Could you check a few things on this model? Use its own coordinates, in mm. A direction names the side the tool comes from. Coordinates: 2 decimals unless noted, no trailing zeros. Loops run counter-clockwise (first coordinate to the right, second up) from the corner with the lowest first, then second, coordinate; pieces in that order, holes last.
1) Imagine slicing it at A-A on x = 0. Please give me the cut outline in (y, z).
2) Will these pins go through, and if not, where does the flat tip stop? P1, Ø3, axis at x = -8, z = 3.5, coming from the -Y side; P2, Ø0.5, axis at y = 0.5, z = 2, coming from the -X side; P3, Ø1.9, axis at x = -11.5, z = 1.5, coming from the -Y side.
3) If I drill on line 1 along Y through (x, z) = (-10.5, 3.1); line 2 along Y through (x, z) = (0, 1.7); line 3 along Z through (x, y) = (16, -1), over which ranges is the centre line in solid material (lowest first)?
4) Imagine slicing it at B-B on x = -10.5. Please give me the cut outline in (y, z), plus the area to 3 significant figures.
5) Thinking about a two-plate mould opening in X: for faces 6 (the face through (8, -3, 5)), 7 (the face through (-9, 1, 2)), 8 (the face through (5.58, 0.1, 2.46)), which applies, released by +X, released by -X, zero draft, split by the parting line, or undercut?
6) For faces 1 (the face through (-7, 0, 2)), 2 (the face through (4.883, -1.928, 3.732)), 3 (the face through (-4.19, 3.16, 3.73)), 4 (the face through (7.98, -0.36, 2.46)), 5 (the face through (3.44, -4.82, 2.46)), which set-ups out of +Z, -Z, +X, -X, +Y, -Y let a thin tool reach every point of the face, with its end or its side?
```python
from build123d import *

# Parameters (mm, degrees)
SKETCH1_R               = 1.5
BOSS_EXTRUDE1_DEPTH     = 5
BOSS_EXTRUDE1_2_DEPTH   = 5
SKETCH1_3_R             = 5.25
BOSS_EXTRUDE2_DEPTH     = 2.5
CUT_EXTRUDE4_DEPTH      = 34.791042337
CUT_EXTRUDE4_DEPTH_BACK = 34.791042337
SKETCH1_5_R             = 3.25
CUT_EXTRUDE1_DEPTH      = 34.791042337
CUT_EXTRUDE2_DEPTH      = 34.791042337
LPATTERN1_COUNT         = 28
LPATTERN1_PITCH         = 0.5
CUT_EXTRUDE3_DEPTH      = 34.791042337
CIRPATTERN1_COUNT       = 8
CIRPATTERN1_ANGLE       = 42


with BuildPart() as part:
    # Sketch1 → Boss-Extrude1 (new body)
    with BuildSketch(Plane.XY):
        with BuildLine():
            Line((-1.559459186, 5.819980914), (-9.630372069, 7.89024295))
            ThreePointArc((-9.630372069, 7.89024295), (-13.619847961, 6.086363356), (-12.727105745, 1.8))
            Line((-12.727105745, 1.8), (-9, 1.8))
            Line((-9, 1.8), (-9, 0))
            Line((-9, 0), (-5.25, 0))
            ThreePointArc((-5.25, 0), (-4.165105037, 3.195997502), (-1.358799987, 5.071110588))
            Line((-1.358799987, 5.071110588), (-1.559459186, 5.819980914))
        make_face()
        with Locations((-10.5, 4.5)):
            Circle(SKETCH1_R, mode=Mode.SUBTRACT)
    extrude(amount=BOSS_EXTRUDE1_DEPTH)



with BuildPart() as body_2:
    # Sketch1 → Boss-Extrude1 2 (new body)
    with BuildSketch(Plane.XY):
        with BuildLine():
            Line((5.983025461, -0.728942102), (5.162088265, 0.956736509))
            ThreePointArc((5.162088265, 0.956736509), (4.867715236, -1.966684615), (3.048690517, -4.274106471))
            Line((3.048690517, -4.274106471), (3.844408913, -5.389662519))
            Line((3.844408913, -5.389662519), (13.676957988, -3.567307264))
            Line((13.676957988, -3.567307264), (32.08570782, 4.250488438))
            Line((32.08570782, 4.250488438), (32.44741195, 6.013772341))
            Line((32.44741195, 6.013772341), (18.681843244, 3.462474984))
            ThreePointArc((18.681843244, 3.462474984), (14.653100202, 0.834635979), (9.916045092, 0))
            Line((9.916045092, 0), (5.983025461, -0.728942102))
        make_face()
    extrude(amount=BOSS_EXTRUDE1_2_DEPTH)


with BuildPart() as part_1:
    add(part.part)

    add(body_2.part)  # Boss-Extrude2 merges body 2
    # Sketch1<3> → Boss-Extrude2 (add)
    with BuildSketch(Plane.XY):
        Circle(SKETCH1_3_R)
    extrude(amount=BOSS_EXTRUDE2_DEPTH)

    # Sketch1<5> → Cut-Extrude4 (cut, two sides: drawn at the far end of the back side and taken through both)
    with BuildSketch(Plane.XY.offset(-CUT_EXTRUDE4_DEPTH_BACK)):
        Circle(SKETCH1_5_R)
    extrude(amount=CUT_EXTRUDE4_DEPTH + CUT_EXTRUDE4_DEPTH_BACK, mode=Mode.SUBTRACT)

    # Sketch2 → Cut-Extrude1 (cut, through all)
    with BuildSketch(Plane(origin=(0, 0, 0), x_dir=(0.9832549075639557, 0.18223552549214142, 0), z_dir=(-0.18223552549214142, 0.9832549075639557, 0))):
        Polygon((13, 0), (33, -1.875), (33, 0), align=None)
        Polygon((33, -3.125), (33, -5), (13, -5), align=None)
    extrude(amount=-CUT_EXTRUDE1_DEPTH, mode=Mode.SUBTRACT)

    # Sketch3 → Cut-Extrude2 (cut, symmetric)
    with BuildSketch(Plane.XY):
        Polygon((31.759133514, 5.886207473), (32.03228257, 5.784278119), (32.250760968, 5.977325236), align=None)
    cut_extrude2 = extrude(amount=CUT_EXTRUDE2_DEPTH, both=True, mode=Mode.SUBTRACT)

    # LPattern1: Cut-Extrude2 ×28
    with Locations(*[Vector(-0.983254907563956, -0.1822355254921403, 0) * (i * LPATTERN1_PITCH) for i in range(1, LPATTERN1_COUNT)]):
        add(cut_extrude2, mode=Mode.SUBTRACT)

    # Sketch4 → Cut-Extrude3 (cut, through all)
    with BuildSketch(Plane.XY):
        Polygon((9.916045092, 0), (11.165663009, 0.030904073), (10.553215679, -0.48439513), align=None)
    cut_extrude3 = extrude(amount=CUT_EXTRUDE3_DEPTH, mode=Mode.SUBTRACT)

    # CirPattern1: Cut-Extrude3 ×8 about axis
    cirpattern1_axis = Axis((10.244577616, 11.995501923, 0), (0, 0, 1))
    for i in range(1, CIRPATTERN1_COUNT):
        add(cut_extrude3.rotate(cirpattern1_axis, i * CIRPATTERN1_ANGLE / (CIRPATTERN1_COUNT - 1)), mode=Mode.SUBTRACT)


solid = part_1.part
```
Filled in:
1. outline: (-5.25, 0) - (-3.25, 0) - (-3.25, 2.5) - (-5.25, 2.5) - close; (3.25, 0) - (5.25, 0) - (5.25, 2.5) - (3.25, 2.5) - close
2. P1: stops at y = 0
2. P2: stops at x = -9
2. P3: stops at y = 1.8
3. line 1: y = 1.8 to 3, 6 to 8
3. line 2: y = -5.25 to -3.25, 3.25 to 5.25
3. line 3: z = 0.24 to 4.76
4. outline: (1.8, 0) - (3, 0) - (3, 5) - (1.8, 5) - close; (6, 0) - (8, 0) - (8, 5) - (6, 5) - close
4. area: 16.0 mm2
5. face 6: zero draft
5. face 7: released by -X
5. face 8: undercut
6. face 1: +Z, -Z, -X, -Y
6. face 2: +Z
6. face 3: +Z, -Y
6. face 4: +Z, -Z, +Y
6. face 5: +Z, -Z, -Y
